Check sheet for the modelled part. Datum: model origin and axes. Units: mm. A direction names the side the tool comes from. Round coordinates to 2 decimals unless told otherwise and drop trailing zeros. Loops run counter-clockwise (first coordinate to the right, second up) from the corner with the lowest first, then second, coordinate; pieces in that order, holes last. Notation, with made-up numbers: (-14, 15) -> (26, 15) arc R27 cw to (26, 38) -> close; hole circle Ø1 at (-37.5, 66). An arc over 180 degrees is marked (long way). Return JSON: item names as keys, results as strings.
from build123d import *

# Parameters (mm, degrees)
F0_R      = 15
F1_DEPTH  = 30
F2_R      = 7.6
F3_DEPTH  = 15
F4_R      = 3.1
F5_DEPTH  = 25.4
F7_DEPTH  = 50.8
F9_DEPTH  = 15.001
F10_R     = 1.8
F11_DEPTH = 25.4


with BuildPart() as f1:
    # F0 (on Top) → F1 (new body)
    with BuildSketch(Plane.XY):
        Circle(F0_R)
    extrude(amount=F1_DEPTH)

    # F2 (on face) → F3 (cut)
    with BuildSketch(Plane.XY.offset(30)):
        Circle(F2_R)
    extrude(amount=-F3_DEPTH, mode=Mode.SUBTRACT)

    # F4 (on face) → F5 (cut)
    with BuildSketch(Plane(origin=(0, 0, 0), x_dir=(1, 0, 0), z_dir=(0, 0, -1))):
        Circle(F4_R)
    extrude(amount=-F5_DEPTH, mode=Mode.SUBTRACT)

    # F6 (on face) → F7 (cut)
    with BuildSketch(Plane(origin=(0, 0, 0), x_dir=(1, 0, 0), z_dir=(0, 0, -1))):
        with BuildLine():
            Line((-1, -14.9666295471), (-1, -19.5340905339))
            Line((-1, -19.5340905339), (1, -19.5340905339))
            Line((1, -19.5340905339), (1, -14.9666295471))
            ThreePointArc((1, -14.9666295471), (0, -15), (-1, -14.9666295471))
        make_face()
        with BuildLine():
            Line((-1, 0), (-1, -2.9342801502))
            ThreePointArc((-1, -2.9342801502), (0, -3.1), (1, -2.9342801502))
            Line((1, -2.9342801502), (1, 0))
            Line((1, 0), (-1, 0))
        make_face()
        with BuildLine():
            Line((-1, -2.9342801502), (-1, -14.9666295471))
            ThreePointArc((-1, -14.9666295471), (0, -15), (1, -14.9666295471))
            Line((1, -14.9666295471), (1, -2.9342801502))
            ThreePointArc((1, -2.9342801502), (0, -3.1), (-1, -2.9342801502))
        make_face()
    extrude(amount=-F7_DEPTH, mode=Mode.SUBTRACT)

    # F8 (on Right) → F9 (cut, through all)
    with BuildSketch(Plane.YZ):
        with BuildLine():
            Line((10.4761691764, 8.6763631552), (10.4761691764, 6.8763631552))
            ThreePointArc((10.4761691764, 6.8763631552), (11.7489613825, 7.4035709491), (12.2761691764, 8.6763631552))
            ThreePointArc((12.2761691764, 8.6763631552), (11.7489613825, 9.9491553614), (10.4761691764, 10.4763631552))
            Line((10.4761691764, 10.4763631552), (10.4761691764, 8.6763631552))
        make_face()
        with BuildLine():
            ThreePointArc((10.4761691764, 10.4763631552), (9.2033769703, 9.9491553614), (8.6761691764, 8.6763631552))
            Line((8.6761691764, 8.6763631552), (10.4761691764, 8.6763631552))
            Line((10.4761691764, 8.6763631552), (10.4761691764, 10.4763631552))
        make_face()
        with BuildLine():
            ThreePointArc((8.6761691764, 8.6763631552), (9.2033769703, 7.4035709491), (10.4761691764, 6.8763631552))
            Line((10.4761691764, 6.8763631552), (10.4761691764, 8.6763631552))
            Line((10.4761691764, 8.6763631552), (8.6761691764, 8.6763631552))
        make_face()
        with BuildLine():
            ThreePointArc((12.2761691764, 21.3597174734), (9.2033769703, 22.6325096795), (10.4761691764, 19.5597174734))
            ThreePointArc((10.4761691764, 19.5597174734), (11.7489613825, 20.0869252673), (12.2761691764, 21.3597174734))
        make_face()
    extrude(amount=-F9_DEPTH, mode=Mode.SUBTRACT)

    # F10 (on face) → F11 (cut)
    with BuildSketch(Plane.YZ.offset(-1)):
        with Locations((10.4761691764, 8.6763631552)):
            Circle(F10_R)
        with Locations((10.4761691764, 21.3597174734)):
            Circle(F10_R)
    extrude(amount=F11_DEPTH, mode=Mode.SUBTRACT)


solid = f1.part
Q1. Section check B-B (x = 7). Record the boundary of the cut face in (y, z), then the cut area to 3 significant figures.
Results list:
{"outline": "(-13.27, 0) -> (13.27, 0) -> (13.27, 30) -> (2.96, 30) -> (2.96, 15) -> (-2.96, 15) -> (-2.96, 30) -> (-13.27, 30) -> close; hole circle Ø3.6 at (10.48, 8.68); hole circle Ø3.6 at (10.48, 21.36)", "area": "687 mm^2"}
Q2. Material ranges on line 1 (X direction, y = 10, z = 23.5); line 2 (X direction, y = 0, z = 9.5); line 3 (Z direction, x = -3.5, y = -1), recorded low to high.
Results list:
{"line 1": "-11.18 to -1, 1 to 11.18", "line 2": "-15 to -3.1, 3.1 to 15", "line 3": "0 to 15"}
Q3. Section check C-C (z = 4.5). Record the boundary of the cut face in (x, y).
Results list:
{"outline": "(-1, 2.93) -> (-1, 14.97) arc R15 ccw (long way) to (1, 14.97) -> (1, 2.93) arc R3.1 cw (long way) to start"}
Q4. Draft check along Y on faces 4 (the flat face through (-1, 10, 11)), 5 (the flat face through (-0.1, -3.3, 15)). Enter one of: released by +Y, released by -Y, zero draft, split by the parting line, or undercut.
Results list:
{"face 4": "zero draft", "face 5": "undercut"}
Q5. Tool access check on faces 1 (the cylindrical face through (-0.32, -7.593, 22.605)), 2 (the flat face through (-7, 4, 30)), 3 (the flat face through (1, 9, 15)). Record the directions out of +Z, -Z, +X, -X, +Y, -Y that give a thin tool (end or side, any length) a straight path to the whole face; none if there is none.
Results list:
{"face 1": "+Z", "face 2": "+Z, +X, -X, +Y, -Y", "face 3": "+Z, -Z, +Y"}
Q6. Section check A-A (y = 8). Record the boundary of the cut face in (x, z), then the cut area to 3 significant figures.
Results list:
{"outline": "(-12.69, 0) -> (-1, 0) -> (-1, 30) -> (-12.69, 30) -> close; (1, 0) -> (12.69, 0) -> (12.69, 30) -> (1, 30) -> close", "area": "701 mm^2"}
Q7. Section check D-D (x = 0). Record the boundary of the cut face in (y, z).
Results list:
{"outline": "(-15, 0) -> (-3.1, 0) -> (-3.1, 15) -> (-7.6, 15) -> (-7.6, 30) -> (-15, 30) -> close"}
Q8. Go/stop test with flat-tipped pins: pin 1 (6 mm diameter, centred on y = 10.48, z = 8.68, fed in from +X); pin 2 (1 mm diameter, centred on x = -9, z = 5, fed in from +Y); pin 3 (5 mm diameter, centred on x = -6.5, z = 25.5, fed in from +Y). Record where each tip stops, or that it passes through.
Results list:
{"pin 1": "x = 13", "pin 2": "y = 12.36", "pin 3": "y = 14.46"}
